from build123d import *

# Parameters (mm, degrees)
SKETCH1_W           = 80
SKETCH1_H           = 12.7
SKETCH1_R           = 2.5
SKETCH1_R_2         = 2
BOSS_EXTRUDE1_DEPTH = 12.7
CUT_EXTRUDE1_DEPTH  = 44.847234804


with BuildPart() as part:
    # Sketch1 → Boss-Extrude1 (new body)
    with BuildSketch(Plane(origin=(0, 0, 0), x_dir=(1, 0, 0), z_dir=(0, 1, 0))):
        Rectangle(SKETCH1_W, SKETCH1_H)
        with Locations(Location((-35, 0, 0), (0, 0, 270))):
            Circle(SKETCH1_R, mode=Mode.SUBTRACT)
        with Locations(Location((-20, 0, 0), (0, 0, 270))):
            Circle(SKETCH1_R, mode=Mode.SUBTRACT)
        with Locations(Location((20, 0, 0), (0, 0, 270))):
            Circle(SKETCH1_R_2, mode=Mode.SUBTRACT)
        with Locations(Location((35, 0, 0), (0, 0, 270))):
            Circle(SKETCH1_R_2, mode=Mode.SUBTRACT)
    extrude(amount=BOSS_EXTRUDE1_DEPTH)

    # Sketch2 → Cut-Extrude1 (cut, through all)
    with BuildSketch(Plane.XY.offset(6.35)):
        with BuildLine():
            ThreePointArc((-1.66625, 8.213762575), (-12.65, 6.35), (-1.66625, 4.486237425))
            ThreePointArc((-1.66625, 4.486237425), (0, 3.85), (1.66625, 4.486237425))
            ThreePointArc((1.66625, 4.486237425), (12.65, 6.35), (1.66625, 8.213762575))
            ThreePointArc((1.66625, 8.213762575), (0, 8.85), (-1.66625, 8.213762575))
        make_face()
    extrude(amount=-CUT_EXTRUDE1_DEPTH, mode=Mode.SUBTRACT)


solid = part.part
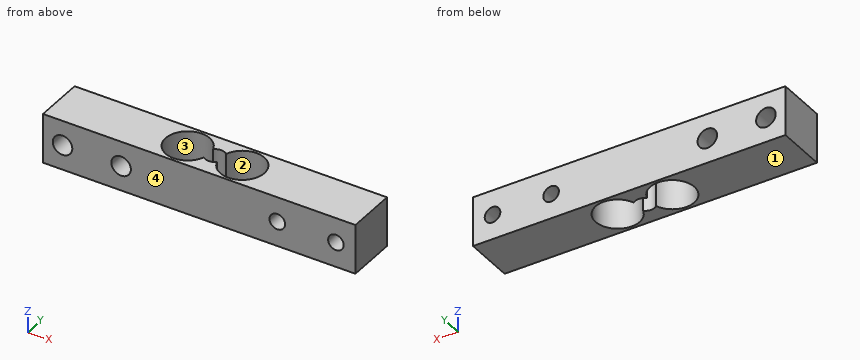
The listing builds one solid part. Answer for the finished solid, in the listing's coordinates (mm). Face numbers are marked on the shaded views. Coordinates: 2 decimals unless noted, no trailing zeros. Write each loop counter-clockwise with the first axis right and the second up, starting at its lowest first coordinate (ties: lowest second). Pieces come first, ordered by that corner, then holes. Notation, with made-up numbers: (88, 24.25) - (95, 24.25) arc R21 cw to (95, 59.25) - close; hole circle Ø11 at (-6, -11). An arc over 180 degrees is marked (long way). Return JSON: item names as keys, results as strings.
1. The part is cut by section C-C on z = 5. Determine the outline of the cut face in (x, y), then the cut area to 3 significant figures.
Final values:
{"outline": "(-40, 0) - (40, 0) - (40, 12.7) - (-40, 12.7) - close; hole (-1.67, 4.49) arc R2.5 ccw to (1.67, 4.49) arc R5.65 ccw (long way) to (1.67, 8.21) arc R2.5 ccw to (-1.67, 8.21) arc R5.65 ccw (long way) to start", "area": "802 mm^2"}
2. The part is cut by section A-A on z = 0. Determine the outline of the cut face in (x, y), then the cut area to 3 significant figures.
Final values:
{"outline": "(-40, 0) - (-37.5, 0) - (-37.5, 12.7) - (-40, 12.7) - close; (-32.5, 0) - (-22.5, 0) - (-22.5, 12.7) - (-32.5, 12.7) - close; (-17.5, 0) - (18, 0) - (18, 12.7) - (-17.5, 12.7) - close; (22, 0) - (33, 0) - (33, 12.7) - (22, 12.7) - close; (37, 0) - (40, 0) - (40, 12.7) - (37, 12.7) - close; hole (-1.67, 4.49) arc R2.5 ccw to (1.67, 4.49) arc R5.65 ccw (long way) to (1.67, 8.21) arc R2.5 ccw to (-1.67, 8.21) arc R5.65 ccw (long way) to start", "area": "573 mm^2"}
3. The part is cut by section D-D on y = 1.5. Determine the outline of the cut face in (x, z).
Final values:
{"outline": "(-40, -6.35) - (-9.9, -6.35) - (-9.9, 6.35) - (-40, 6.35) - close; (-4.1, -6.35) - (4.1, -6.35) - (4.1, 6.35) - (-4.1, 6.35) - close; (9.9, -6.35) - (40, -6.35) - (40, 6.35) - (9.9, 6.35) - close; hole circle Ø5 at (-35, 0); hole circle Ø5 at (-20, 0); hole circle Ø4 at (20, 0); hole circle Ø4 at (35, 0)"}
4. The part is cut by section B-B on x = -7. Determine the outline of the cut face in (y, z), then the cut area to 3 significant figures.
Final values:
{"outline": "(0, -6.35) - (0.7, -6.35) - (0.7, 6.35) - (0, 6.35) - close; (12, -6.35) - (12.7, -6.35) - (12.7, 6.35) - (12, 6.35) - close", "area": "17.8 mm^2"}
5. For a pull along Y with two mould halves and no side action, classify the marked faces 1, 2, 3 and 4 as +Y half, -Y half, draft (parallel to the pull), parting line (faces both ways), or undercut.
Final values:
{"face 1": "draft", "face 2": "undercut", "face 3": "undercut", "face 4": "-Y half"}
6. This flat-tipped pin is pushed along its axis until it touches: pin 1 Ø4.5 at (x, z) = (-35, 0) entering from -Y. Where does it stop, or does it pass through?
Final values:
{"pin 1": "through"}
7. Consider line 1 along Y through (x, z) = (7, -1); line 2 along X through (y, z) = (6.25, -3.75); line 3 along X through (y, z) = (7, 0). Determine where each line is inside the solid, lowest interval first.
Final values:
{"line 1": "0 to 0.7, 12 to 12.7", "line 2": "-40 to -12.65, 12.65 to 40", "line 3": "-40 to -37.5, -32.5 to -22.5, -17.5 to -12.61, 12.61 to 18, 22 to 33, 37 to 40"}
